Check sheet for the modelled part. Datum: model origin and axes. Units: mm. Round coordinates to 2 decimals unless told otherwise and drop trailing zeros. Order: outer loops, then holes, each group sorted by start corner. A loop starts at its lowest first (then second) coordinate and runs counter-clockwise, first axis right, second up. Notation, with made-up numbers: (-9, -13) -> (-1, -13) arc R19 ccw to (-1, 6) -> close; hole circle Ø3 at (-9.5, 0.5). An arc over 180 degrees is marked (long way). Answer in a Markdown table with one row per item.
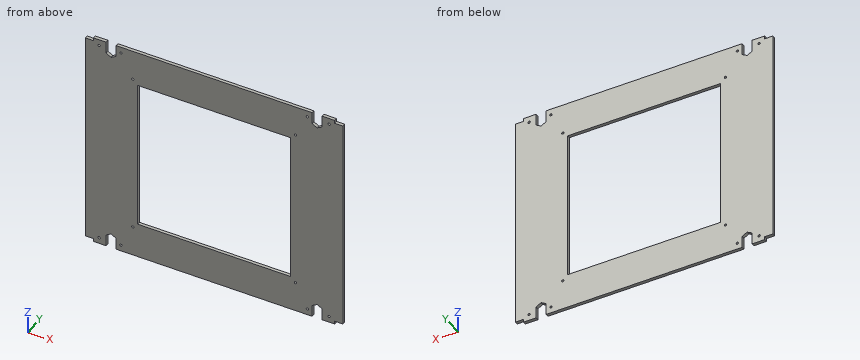
from build123d import *

# Parameters (mm, degrees)
SKETCH1_R           = 1.5
SKETCH1_W           = 196.314766664
SKETCH1_H           = 196.314766664
BOSS_EXTRUDE1_DEPTH = 4


with BuildPart() as part:
    # Sketch1 → Boss-Extrude1 (new body)
    with BuildSketch(Plane(origin=(0, 0, 0), x_dir=(1, 0, 0), z_dir=(0, 1, 0))):
        Polygon((154.855, -139.95), (165.325, -139.95), (165.325, 139.95), (154.855, 139.95), (154.855, 143.95), (138.875, 143.95), (138.875, 128.61722325), (132.375, 124.864446501), (125.875, 128.61722325), (125.875, 143.95), (-125.875, 143.95), (-125.875, 128.61722325), (-132.375, 124.864446501), (-138.875, 128.61722325), (-138.875, 143.95), (-154.855, 143.95), (-154.855, 139.95), (-165.325, 139.95), (-165.325, -139.95), (-154.855, -139.95), (-154.855, -143.95), (-138.875, -143.95), (-138.875, -128.61722325), (-132.375, -124.864446501), (-125.875, -128.61722325), (-125.875, -143.95), (125.875, -143.95), (125.875, -128.61722325), (132.375, -124.864446501), (138.875, -128.61722325), (138.875, -143.95), (154.855, -143.95), align=None)
        with Locations(Location((-147.795, -135.95, 0), (0, 0, 270))):
            Circle(SKETCH1_R, mode=Mode.SUBTRACT)
        with Locations(Location((-119.795, -135.95, 0), (0, 0, 270))):
            Circle(SKETCH1_R, mode=Mode.SUBTRACT)
        with Locations(Location((-104.5, -104.5, 0), (0, 0, 270))):
            Circle(SKETCH1_R, mode=Mode.SUBTRACT)
        with Locations(Location((119.795, -135.95, 0), (0, 0, 270))):
            Circle(SKETCH1_R, mode=Mode.SUBTRACT)
        with Locations(Location((147.795, -135.95, 0), (0, 0, 270))):
            Circle(SKETCH1_R, mode=Mode.SUBTRACT)
        with Locations(Location((104.5, -104.5, 0), (0, 0, 270))):
            Circle(SKETCH1_R, mode=Mode.SUBTRACT)
        with Locations(Location((-104.5, 104.5, 0), (0, 0, 270))):
            Circle(SKETCH1_R, mode=Mode.SUBTRACT)
        with Locations(Location((-147.795, 135.95, 0), (0, 0, 270))):
            Circle(SKETCH1_R, mode=Mode.SUBTRACT)
        with Locations(Location((-119.795, 135.95, 0), (0, 0, 270))):
            Circle(SKETCH1_R, mode=Mode.SUBTRACT)
        Rectangle(SKETCH1_W, SKETCH1_H, mode=Mode.SUBTRACT)
        with Locations(Location((104.5, 104.5, 0), (0, 0, 270))):
            Circle(SKETCH1_R, mode=Mode.SUBTRACT)
        with Locations(Location((119.795, 135.95, 0), (0, 0, 270))):
            Circle(SKETCH1_R, mode=Mode.SUBTRACT)
        with Locations(Location((147.795, 135.95, 0), (0, 0, 270))):
            Circle(SKETCH1_R, mode=Mode.SUBTRACT)
    extrude(amount=BOSS_EXTRUDE1_DEPTH)


solid = part.part
Item 1: Cross-section at C-C (y = 0.8). State how many separate pieces and enclosed holes the cut face has, and give its area (3 significant figures).
Result sheet:
| item | result |
|---|---|
| separate pieces | 1 |
| enclosed holes | 13 |
| area | 55,500 mm^2 |
Item 2: Scan lines: line 1 (Z direction, x = -63.5, y = 1.95); line 2 (X direction, y = 1.35, z = 35) (3 decimals); line 3 (X direction, y = 1.8, z = 104.5) (3 decimals). Record each from-to range of solid material in increasing order. Write a range as [from, to].
Result sheet:
| item | result |
|---|---|
| line 1 | z = [-143.95, -98.16], [98.16, 143.95] |
| line 2 | x = [-165.325, -98.157], [98.157, 165.325] |
| line 3 | x = [-165.325, -106], [-103, 103], [106, 165.325] |
Item 3: Depth check by flat-ended pin: P1, Ø1.2, axis at y = 2.5, z = 142, coming from the +X side (3 decimals). Enter the tip coordinate at first touch or a pass-through.
Result sheet:
| item | result |
|---|---|
| P1 | stops at x = 154.855 |
Item 4: Cross-section at A-A (x = -75.5). Record the boundary of the cut face in (y, z).
Result sheet:
| item | result |
|---|---|
| outline | (0, -143.95) -> (4, -143.95) -> (4, -98.16) -> (0, -98.16) -> close; (0, 98.16) -> (4, 98.16) -> (4, 143.95) -> (0, 143.95) -> close |
Item 5: Cross-section at B-B (z = -56). Record the boundary of the cut face in (x, y) (3 decimals), and give its area (3 significant figures).
Result sheet:
| item | result |
|---|---|
| outline | (-165.325, 0) -> (-98.157, 0) -> (-98.157, 4) -> (-165.325, 4) -> close; (98.157, 0) -> (165.325, 0) -> (165.325, 4) -> (98.157, 4) -> close |
| area | 537 mm^2 |
